Verification items for the finished model (mm, model axes). Face numbers are marked on the shaded views. A direction names the side the tool comes from. Give positions to 0.01 mm unless a question says otherwise; leave off trailing zeros. Order: outer loops, then holes, each group sorted by start corner. A loop starts at its lowest first (then second) coordinate and runs counter-clockwise, first axis right, second up. Notation, with made-up numbers: (4.25, 21) -> (28.25, 21) arc R14 cw to (28.25, 36) -> close; hole circle Ø10 at (31.25, -32.75). An arc over 180 degrees is marked (long way). Write each question's results on one line, items separated by ' | '. Start each with the question number.
1. Cross-section at D-D, the plane y = -10.5. Enter the section's corners in (x, z).
2. Cross-section at C-C, the plane z = -58.5. Enter the section's corners in (x, y).
3. Set-up check for the marked faces 1 and 2: record each of +Z, -Z, +X, -X, +Y, -Y from which the full face is reachable in a straight line by a thin tool's end or side.
4. Mould release check, pull along X, two halves, no side actions. Record for the marked faces 3, 4, 5 and 6: +X half, -X half, draft (parallel to the pull), parting line (faces both ways), or undercut.
5. Depth check by flat-ended pin: pin 1 Ø1 at (x, y) = (133.5, 20) entering from -Z; pin 2 Ø8 at (x, y) = (83, 5) entering from -Z. Enter the tip coordinate at first touch or a pass-through.
6. Cross-section at A-A, the plane x = 40.5. Enter the section's corners in (y, z).
7. Material ranges on L1, parallel to Y at x = -8.8, z = -67.5; L2, parallel to Z at x = -8.1, y = 77; L3, parallel to X at y = 26.5, z = -18, recorded low to high. Write a range as from..to.
8. Cross-section at B-B, the plane z = -48.5. Enter the section's corners in (x, y), then the cut area to 3 significant figures.
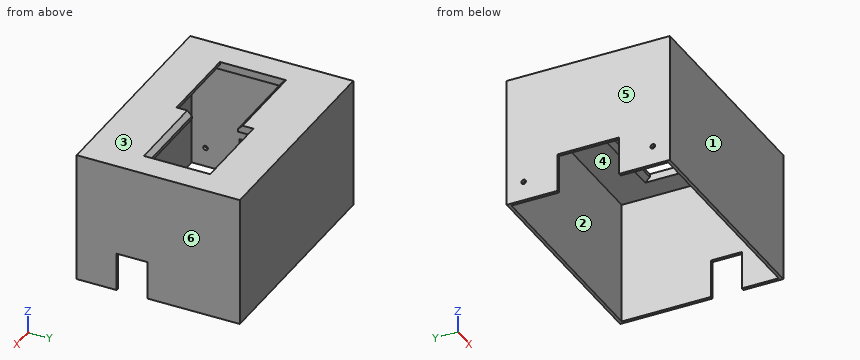
Autodesk Inventor part; units mm, degrees
ref_plane "YZ Plane" through (0, 0, 0) normal (1, 0, 0) x (0, 1, 0)
ref_plane "XZ Plane" through (0, 0, 0) normal (0, 1, 0) x (-1, 0, 0)
ref_plane "XY Plane" through (0, 0, 0) normal (0, 0, 1) x (1, 0, 0)
sketch "Sketch1" plane through (0, 0, 0) normal (0, 0, 1) x (1, 0, 0)
  line L0 (0, 0) -> (0, 70) construction
  circle A0 centre (0, 0) radius 2.5
  circle A1 centre (0, 70) radius 2.5
  line L1 (0, 0) -> (125, 0) construction
  circle A2 centre (125, 0) radius 2.5
  circle A3 centre (125, 70) radius 2.5
  line L2 (-7.5, -16) -> (132.5, -16)
  line L3 (132.5, -16) -> (132.5, 86)
  line L4 (132.5, 86) -> (-7.5, 86)
  line L5 (-7.5, 86) -> (-7.5, -16)
  point P0 (62.5, 0)
  point P1 (62.5, -16)
  point P2 (0, 35)
  point P3 (-7.5, 35)
  dimension "d0" = 70
  dimension "d1" = 5
  dimension "d2" = 5
  dimension "d3" = 5
  dimension "d4" = 5
  dimension "d5" = 125
  dimension "d6" = 140
  dimension "d7" = 102
extrude "Extrusion1" add sketch "Sketch1" along normal blind 5
sketch "Sketch2" plane through (0, 0, 5) normal (0, 0, 1) x (1, 0, 0)
  line L0 (7.5, 60) -> (117.5, 60)
  line L1 (117.5, 60) -> (117.5, 10)
  line L2 (117.5, 10) -> (7.5, 10)
  line L3 (7.5, 10) -> (7.5, 60)
  line L4 (-7.5, 86) -> (-7.5, -16)
  line L5 (132.5, 86) -> (-7.5, 86)
  point P0 (0, 0)
  point P1 (62.5, 60)
  point P2 (62.5, 86)
  point P3 (7.5, 35)
  point P4 (-7.5, 35)
  dimension "d10" = 15
  dimension "d11" = 50
extrude "Extrusion2" cut sketch "Sketch2" against normal through all
sketch "Sketch3" plane through (-7.5, 86, 0) normal (0, 1, 0) x (1, 0, 0)
  line L0 (140, 0) -> (140, -5)
  line L1 (140, -5) -> (0, -5)
  line L2 (0, -5) -> (0, 80)
  line L3 (0, 80) -> (140, 80)
  line L4 (140, 80) -> (140, -5)
  point P0 (7.5, 0)
  dimension "d17" = 85
extrude "Extrusion3" add sketch "Sketch3" along normal blind 2
sketch "Sketch4" plane through (-7.5, -16, 0) normal (0, -1, 0) x (1, 0, 0)
  line L0 (140, 0) -> (0, 0)
  line L1 (0, 0) -> (0, -80)
  line L2 (0, -80) -> (140, -80)
  line L3 (140, -80) -> (140, 0)
  line L4 (0, 0) -> (140, 0)
  line L5 (140, 0) -> (140, 5)
  line L6 (0, 5) -> (140, 5)
  line L7 (0, 0) -> (0, 5)
  point P0 (7.5, 0)
extrude "Extrusion4" add sketch "Sketch4" along normal blind 2
sketch "Sketch5" plane through (-7.5, 86, -80) normal (-1, 0, 0) x (0, 0, 1)
  line L0 (85, -104) -> (85, 2)
  line L1 (0, -102) -> (0, -104)
  line L2 (85, 2) -> (0, 2)
  line L3 (0, 2) -> (0, -104)
  line L4 (0, -104) -> (85, -104)
  line L5 (85, -104) -> (85, 2)
  point P0 (80, -86)
extrude "Extrusion5" add sketch "Sketch5" along normal blind 2
sketch "Sketch6" plane through (132.5, 86, 0) normal (1, 0, 0) x (0, 0, -1)
  line L0 (-5, -104) -> (-5, 2)
  line L1 (-5, -104) -> (80, -104)
  line L2 (80, -104) -> (80, 2)
  line L3 (80, 2) -> (-5, 2)
  line L4 (-5, 2) -> (-5, -104)
  point P0 (0, -86)
extrude "Extrusion6" add sketch "Sketch6" along normal blind 2
sketch "Sketch7" plane through (0, 0, 5) normal (0, 0, 1) x (1, 0, 0)
  line L0 (117.5, 10) -> (7.5, 10) construction
  line L1 (7.5, 60) -> (117.5, 60) construction
  line L2 (7.5, 10) -> (7.5, 60) construction
  line L3 (117.5, 60) -> (117.5, 10) construction
  line L4 (7.5, 60) -> (62.5, 60)
  line L5 (62.5, 60) -> (62.5, 50)
  line L6 (62.5, 50) -> (7.5, 50)
  line L7 (7.5, 50) -> (7.5, 60)
  line L8 (117.5, 10) -> (62.5, 10)
  line L9 (62.5, 10) -> (62.5, 20)
  line L10 (62.5, 20) -> (117.5, 20)
  line L11 (117.5, 20) -> (117.5, 10)
  line L12 (117.5, 10) -> (7.5, 10)
  line L13 (7.5, 60) -> (117.5, 60)
  line L14 (7.5, 10) -> (7.5, 60)
  point P0 (0, 0)
  point P1 (62.5, 10)
  point P2 (7.5, 35)
  dimension "d26" = 55
  dimension "d27" = 10
  dimension "d28" = 55
  dimension "d29" = 10
extrude "Extrusion7" add sketch "Sketch7" against normal blind 5
chamfer "Chamfer2" distance 3 angle 45 4 edges at (35, 10, 0) (90, 60, 0) (90, 20, 5) (35, 50, 5)
sketch "Sketch8" plane through (134.5, 86, 0) normal (1, 0, 0) x (0, 0, -1)
  line L0 (80, -104) -> (80, 2)
  line L1 (80, -102) -> (80, 0)
  line L2 (80, -51) -> (93.9386, -51)
  line L3 (80, -78.0836) -> (55, -78.0836)
  line L4 (55, -78.0836) -> (55, -58.0836)
  line L5 (55, -58.0836) -> (80, -58.0836)
  line L6 (80, -58.0836) -> (80, -78.0836)
  point P0 (0, -86)
  dimension "d36" = 20
  dimension "d37" = 25
  dimension "d40" = 7.0836
extrude "Extrusion8" cut sketch "Sketch8" against normal blind 10
sketch "Sketch9" plane through (-9.5, 86, -80) normal (-1, 0, 0) x (0, 0, 1)
  line L0 (0, -58.0836) -> (0, 0)
  line L1 (0, -31) -> (25, -31)
  line L2 (25, -31) -> (25, -71)
  line L3 (25, -71) -> (0, -71)
  line L4 (0, -71) -> (0, -31)
  line L5 (0, 2) -> (0, -104)
  line L6 (0, -71) -> (25, -71)
  line L7 (25, -71) -> (25, -31)
  line L8 (25, -31) -> (0, -31)
  line L9 (0, -31) -> (0, -71)
  point P0 (80, -86)
  point P1 (0, -51)
  dimension "d41" = 40
  dimension "d42" = 25
extrude "Extrusion9" cut sketch "Sketch9" against normal blind 10
sketch "Sketch10" plane through (-9.5, 86, -80) normal (-1, 0, 0) x (0, 0, 1)
  circle A0 centre (12.5, -93) radius 1.5
  circle A1 centre (12.5, -9) radius 1.5
  line L0 (12.5, -93) -> (12.5, -9) construction
  line L1 (85, -104) -> (85, 2)
  line L2 (25, -71) -> (0, -71)
  point P0 (80, -86)
  point P1 (85, -51)
  point P2 (12.5, -51)
  point P3 (12.5, -71)
  point P4 (12.5, -71)
  dimension "d45" = 3
  dimension "d46" = 3
  dimension "d47" = 84
extrude "Extrusion10" cut sketch "Sketch10" against normal blind 10
sketch "Sketch11" plane through (0, 0, 5) normal (0, 0, 1) x (1, 0, 0)
  circle A0 centre (0, 0) radius 2.5
  circle A1 centre (0, 70) radius 2.5
  circle A2 centre (125, 0) radius 2.5
  circle A3 centre (125, 70) radius 2.5
extrude "Extrusion11" add sketch "Sketch11" against normal blind 5
properties part number "GA06" material "ABS Plastic"
Results below:
1) outline: (-9.5, -80) -> (-7.5, -80) -> (-7.5, 0) -> (132.5, 0) -> (132.5, -80) -> (134.5, -80) -> (134.5, 5) -> (-9.5, 5) -> close
2) outline: (-9.5, -18) -> (134.5, -18) -> (134.5, 7.92) -> (132.5, 7.92) -> (132.5, -16) -> (-7.5, -16) -> (-7.5, 15) -> (-9.5, 15) -> close; (-9.5, 55) -> (-7.5, 55) -> (-7.5, 86) -> (132.5, 86) -> (132.5, 27.92) -> (134.5, 27.92) -> (134.5, 88) -> (-9.5, 88) -> close
3) face 1: +Z, -Z, +X, -X, -Y | face 2: -Z
4) face 3: draft | face 4: undercut | face 5: -X half | face 6: +X half
5) pin 1: stops at z = -55 | pin 2: stops at z = 0
6) outline: (-18, -80) -> (-16, -80) -> (-16, 0) -> (7, 0) -> (10, 3) -> (10, 5) -> (-18, 5) -> close; (50, 0) -> (86, 0) -> (86, -80) -> (88, -80) -> (88, 5) -> (53, 5) -> (50, 2) -> close
7) L1: y = -18..-8.5, -5.5..15, 55..75.5, 78.5..88 | L2: z = -80..-69, -66..5 | L3: x = -9.5..-7.5, 132.5..134.5
8) outline: (-9.5, -18) -> (134.5, -18) -> (134.5, 88) -> (-9.5, 88) -> close; hole (-7.5, -16) -> (132.5, -16) -> (132.5, 86) -> (-7.5, 86) -> close | area: 984 mm²
